Job drawing, mm, ordinate dimensions from the low corner. One solid piece. A direction names the side the tool comes from. Coordinates: 2 decimals unless noted, no trailing zeros. Order: outer loops, then holes, each group sorted by start corner. A loop starts at its lowest first (then second) coordinate and runs counter-clockwise, first axis right, second up. Notation, with made-up numbers: M -22.5,32 L 10.5,32 A11 ccw 10.5,42 Z; hole C 68,63.5 d4. An arc over 180 degrees is marked long. Write item = value, one per line. Start each with the question number.
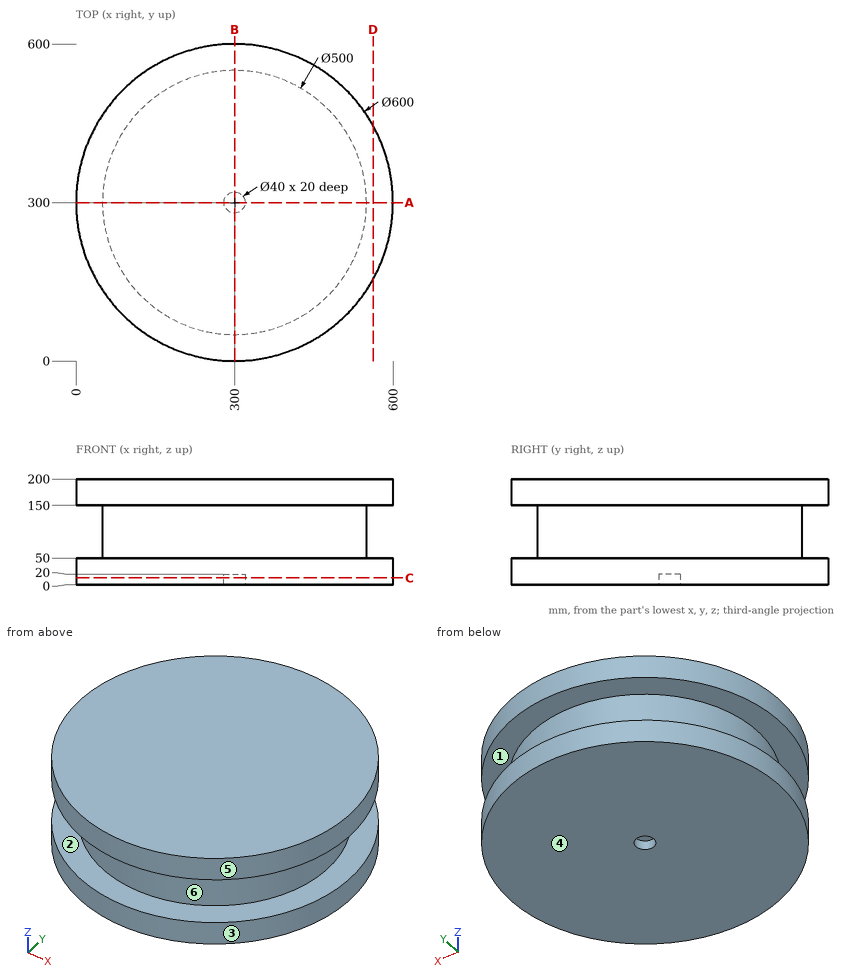
1. Slice it at D-D (x = 562.5). Write the cut outline in (y, z), plus the area to 3 significant figures.
2. Flat gauge pins, fed straight in: pin 1 (12 mm diameter, centred on y = 510.5, z = 33.5, fed in from +X); pin 2 (12 mm diameter, centred on x = 402, z = 157.5, fed in from +Y); pin 3 (2 mm diameter, centred on y = 161.5, z = 135, fed in from -X). Where does each tip first touch, or does it go through?
3. Probe L1, parallel to Y at x = 300, z = 6.5; L2, parallel to Z at x = 491.5, y = 485.5; L3, parallel to X at y = 297.5, z = 71.5. List the from-to ranges inside material, lowest first.
4. Slice it at A-A (y = 300). Write the cut outline in (x, z), plus the area to 3 significant figures.
5. Mould opens along Z. For the marked faces 1, 2, 3 and 4 say: released by +Z, released by -Z, zero draft, split by the parting line, or undercut.
6. Slice it at C-C (z = 13). Write the cut outline in (x, y), plus the area to 3 significant figures.
7. 3-axis set-ups, long thin cutter, end or side, ignore diameter. For the marked faces 5 and 6: which of +Z, -Z, +X, -X, +Y, -Y reach the whole face in a straight line?
Calculated:
q1.outline = M 154.76,0 L 445.24,0 L 445.24,50 L 154.76,50 Z; M 154.76,150 L 445.24,150 L 445.24,200 L 154.76,200 Z
q1.area = 29,000 mm²
q2.pin_1 = 519.5
q2.pin_2 = 584.23
q2.pin_3 = 91.21
q3.L1 = 0 to 280, 320 to 600
q3.L2 = 0 to 50, 150 to 200
q3.L3 = 50.01 to 549.99
q4.outline = M 0,0 L 280,0 L 280,20 L 320,20 L 320,0 L 600,0 L 600,50 L 550,50 L 550,150 L 600,150 L 600,200 L 0,200 L 0,150 L 50,150 L 50,50 L 0,50 Z
q4.area = 109,000 mm²
q5.face_1 = undercut
q5.face_2 = undercut
q5.face_3 = zero draft
q5.face_4 = released by -Z
q6.outline = C 300,300 d600; hole C 300,300 d40
q6.area = 281,000 mm²
q7.face_5 = +Z, -Z
q7.face_6 = none
